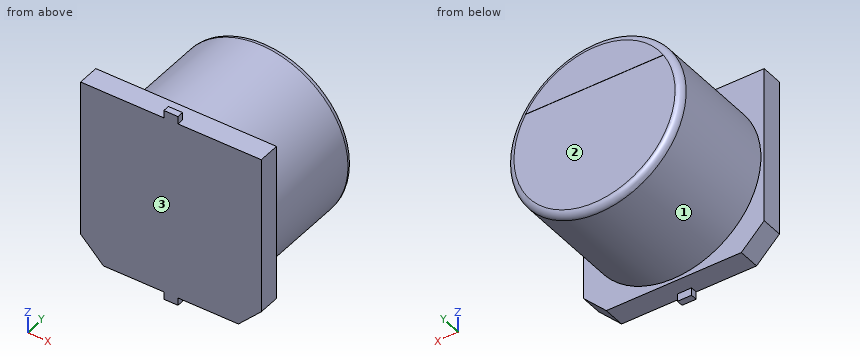
```python
from build123d import *

# Parameters (mm, degrees)
BOSS_EXTRUDE1_DEPTH = 1
SKETCH3_R           = 4
BOSS_EXTRUDE2_DEPTH = 6.2
FILLET1_R           = 0.3
SKETCH4_W           = 0.65
SKETCH4_H           = 3.4
BOSS_EXTRUDE3_DEPTH = 0.3
BOSS_EXTRUDE4_DEPTH = 0.01


with BuildPart() as part:
    # Sketch2 → Boss-Extrude1 (new body)
    with BuildSketch(Plane(origin=(0, 0, 0), x_dir=(1, 0, 0), z_dir=(0, 1, 0))):
        Polygon((4.15, -4.15), (-4.15, -4.15), (-4.15, 3.1), (-3.1, 4.15), (3.1, 4.15), (4.15, 3.1), align=None)
    extrude(amount=BOSS_EXTRUDE1_DEPTH)

    # Sketch3 → Boss-Extrude2 (add)
    with BuildSketch(Plane(origin=(0, 0, 0), x_dir=(1, 0, 0), z_dir=(0, 1, 0))):
        Circle(SKETCH3_R)
    extrude(amount=BOSS_EXTRUDE2_DEPTH)

    # Fillet1
    fillet1_edges = [part.edges().sort_by_distance(p)[0] for p in [
        (-4, 6.2, 0),
    ]]
    fillet(fillet1_edges, radius=FILLET1_R)

    # Sketch4 → Boss-Extrude3 (add)
    with BuildSketch(Plane(origin=(0, 0, 0), x_dir=(1, 0, 0), z_dir=(0, 1, 0))):
        with Locations((0, 2.8)):
            Rectangle(SKETCH4_W, SKETCH4_H)
        with Locations((0, -2.8)):
            Rectangle(SKETCH4_W, SKETCH4_H)
    extrude(amount=BOSS_EXTRUDE3_DEPTH)

    # Sketch5 → Boss-Extrude4 (add)
    with BuildSketch(Plane(origin=(0, 6.2, 0), x_dir=(1, 0, 0), z_dir=(0, 1, 0))):
        with BuildLine():
            Line((-3.165033817, -1.916392689), (3.165033817, -1.916392689))
            ThreePointArc((3.165033817, -1.916392689), (0, -3.7), (-3.165033817, -1.916392689))
        make_face()
    extrude(amount=BOSS_EXTRUDE4_DEPTH)


solid = part.part
```
Geometry: final body of the model. Coordinates: model frame, mm. Face numbers are marked on the shaded views. A direction names the side the tool comes from. Coordinates: 2 decimals unless noted, no trailing zeros. Order: outer loops, then holes, each group sorted by start corner. A loop starts at its lowest first (then second) coordinate and runs counter-clockwise, first axis right, second up. Notation, with made-up numbers: (51, 37.25) -> (74, 37.25) arc R11 cw to (74, 55.25) -> close; hole circle Ø6 at (-39, 30). An arc over 180 degrees is marked (long way). Use CSV: the item, a comma, the result in double quotes.
1) Section C-C on y = 1.5. Output: boundary loops of the cut face in (x, z).
Findings:
outline,"circle Ø8 at (0, 0)"
2) Pin query (flat end, axial travel): pin 1 Ø1.7 at (x, z) = (1.5, -1.5) entering from +Y; pin 2 Ø2 at (x, y) = (-2.5, 2.5) entering from -Z; pin 3 Ø3 at (x, y) = (2.5, 4.5) entering from +Z. Return the tip coordinate at first contact, or that it passes through.
Findings:
pin 1,"stops at y = 6.2"
pin 2,"stops at z = -3.71"
pin 3,"stops at z = 3.87"
3) Access query for the marked faces 1, 2 and 3. Directions: +Z, -Z, +X, -X, +Y, -Y. A direction counts if a zero-diameter tool reaches every point of the face in a straight line with its end or side. Return the directions, or none.
Findings:
face 1,"+Y"
face 2,"-Z, +X, -X, +Y"
face 3,"+Z, -Z, +X, -X, -Y"
4) Line query: line 1 (Y direction, x = 0.5, z = -0.25); line 2 (X direction, y = 4.25, z = 0); line 3 (Y direction, x = 3.75, z = -1.75). Output: solid intervals per line, ascending.
Findings:
line 1,"y = 0 to 6.2"
line 2,"x = -4 to 4"
line 3,"y = 0 to 1"
5) Section A-A on z = 0. Output: boundary loops of the cut face in (x, y).
Findings:
outline,"(-4.15, 0) -> (4.15, 0) -> (4.15, 1) -> (4, 1) -> (4, 5.9) arc R0.3 ccw to (3.7, 6.2) -> (-3.7, 6.2) arc R0.3 ccw to (-4, 5.9) -> (-4, 1) -> (-4.15, 1) -> close"
